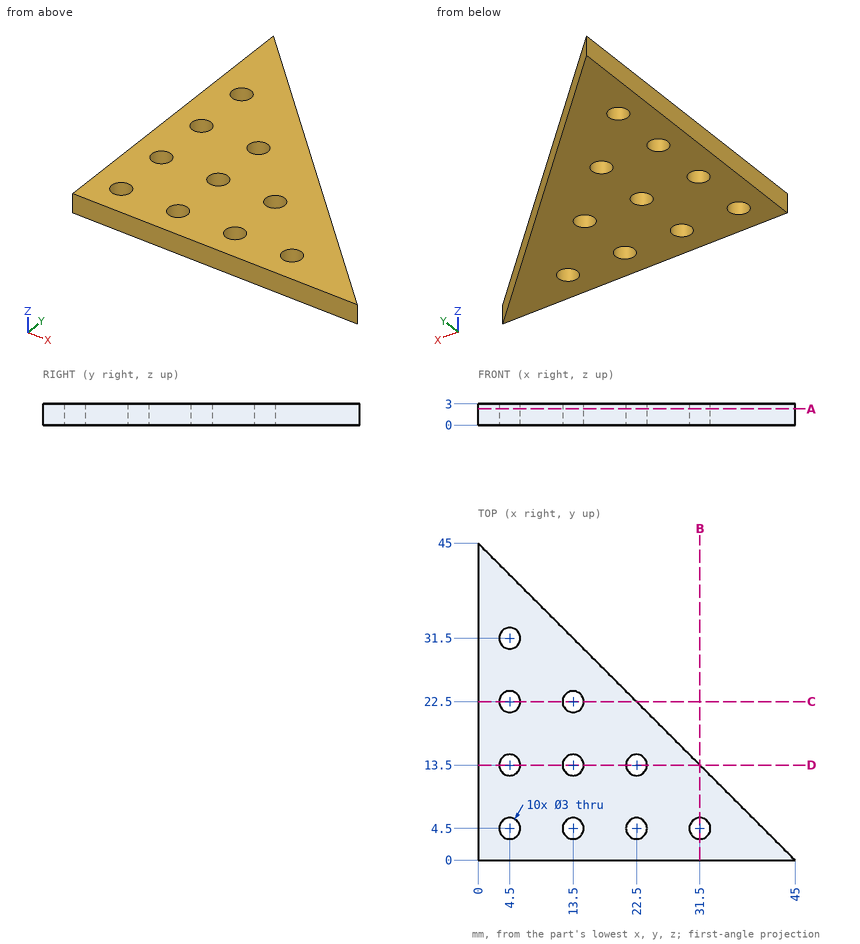
For this review, use the dimensioned drawing (mm, ordinates from the lowest corner) and the shaded views. Coordinates: 2 decimals unless noted, no trailing zeros. Order: outer loops, then holes, each group sorted by start corner. A loop starts at its lowest first (then second) coordinate and runs counter-clockwise, first axis right, second up. Notation, with made-up numbers: (82, -24) - (105, -24) arc R26 ccw to (105, 13) - close; hole circle Ø2 at (84, -15). An arc over 180 degrees is marked (long way). Answer as a JSON object with one key per item and string values. Group by question number.
1. We need section A-A on z = 2.3. Give the number of separate pieces and of enclosed holes in the cut face, then the cut area to 3 significant figures.
2. We need section B-B on x = 31.5. State the section outline as (y, z) points, then the cut area to 3 significant figures.
3. For probe 1 along Y at (x, z) = (22.5, 2.25); probe 2 along Y at (x, z) = (13.5, 1.9); probe 3 along Y at (x, z) = (5, 0.6), list the stretches that pass through material, from the lowest coordinate up.
4. We need section C-C on y = 22.5. State the section outline as (x, z) points.
5. Clearance check with a flat-ended pin moving along its axis: P1, Ø1, axis at x = 28, z = 0.5, coming from the +Y side. State where the tip first meets the part, or that it passes through.
6. We need section D-D on y = 13.5. State the section outline as (x, z) points, then the cut area to 3 significant figures.
Final values:
{
 "1": {"separate pieces": "1", "enclosed holes": "10", "area": "942 mm²"},
 "2": {"outline": "(0, 0) - (3, 0) - (3, 3) - (0, 3) - close; (6, 0) - (13.5, 0) - (13.5, 3) - (6, 3) - close", "area": "31.5 mm²"},
 "3": {"probe 1": "0 to 3, 6 to 12, 15 to 22.5", "probe 2": "0 to 3, 6 to 12, 15 to 21, 24 to 31.5", "probe 3": "0 to 3.09, 5.91 to 12.09, 14.91 to 21.09, 23.91 to 30.09, 32.91 to 40"},
 "4": {"outline": "(0, 0) - (3, 0) - (3, 3) - (0, 3) - close; (6, 0) - (12, 0) - (12, 3) - (6, 3) - close; (15, 0) - (22.5, 0) - (22.5, 3) - (15, 3) - close"},
 "5": {"P1": "y = 17.5"},
 "6": {"outline": "(0, 0) - (3, 0) - (3, 3) - (0, 3) - close; (6, 0) - (12, 0) - (12, 3) - (6, 3) - close; (15, 0) - (21, 0) - (21, 3) - (15, 3) - close; (24, 0) - (31.5, 0) - (31.5, 3) - (24, 3) - close", "area": "67.5 mm²"}
}
